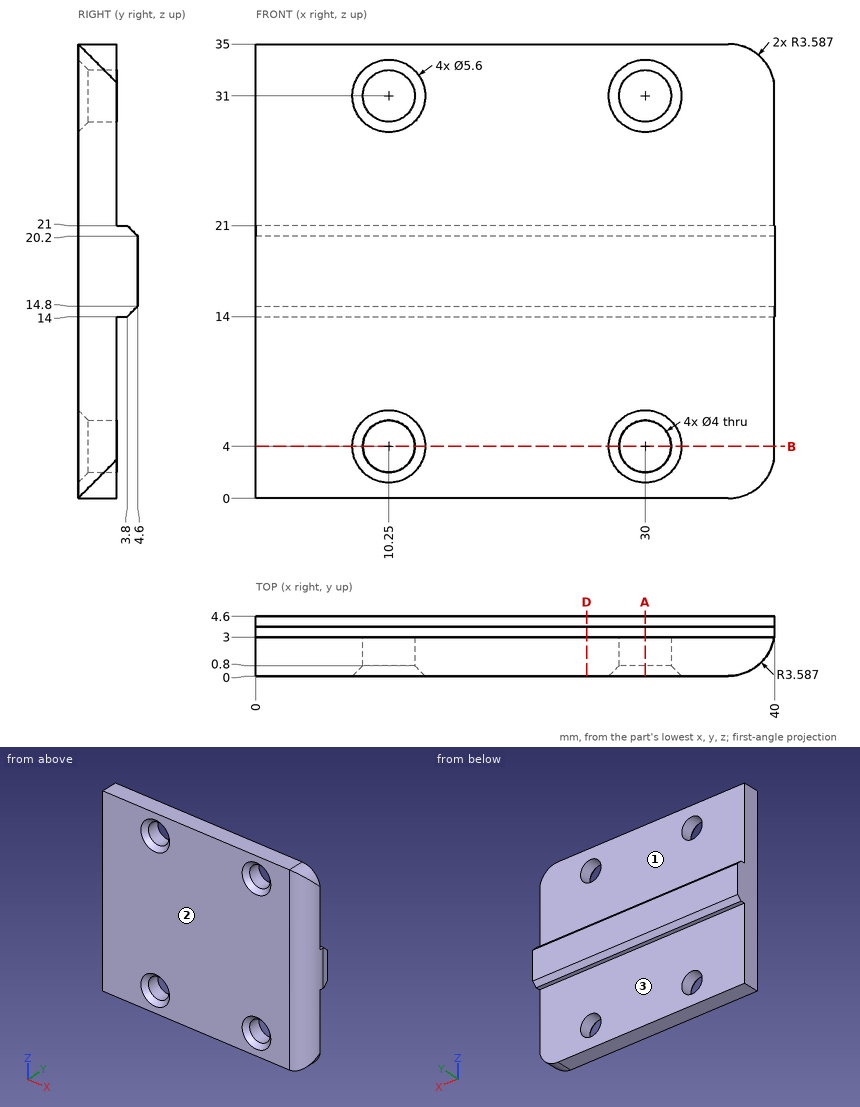
Geometry: see drawing. Coordinates: mm, zero at the bounding-box minimum. A direction names the side the tool comes from. Round coordinates to 2 decimals unless told otherwise and drop trailing zeros. Loops run counter-clockwise (first coordinate to the right, second up) from the corner with the lowest first, then second, coordinate; pieces in that order, holes last. Notation, with made-up numbers: M 41.5,89 L 69.5,89 A21 cw 69.5,115 Z; hole C 53,34 d8. An arc over 180 degrees is marked long. Use a Markdown table: item, result. Add a question column.
1. Cut plane D-D, the plane x = 25.5. Output: boundary loops of the cut face in (y, z).
2. Contact query for flat-ended pins moving along their axis: pin 1 (4.5 mm diameter, centred on x = 30, z = 4, fed in from +Y); pin 2 (2 mm diameter, centred on x = 7.5, y = 1.5, fed in from -Z); pin 3 (3.5 mm diameter, centred on x = 10.25, z = 4, fed in from +Y); pin 4 (2 mm diameter, centred on y = 1.5, z = 5, fed in from +X). Output: stop coordinate, or through.
3. Cut plane B-B, the plane z = 4. State how many separate pieces and enclosed holes the cut face has.
4. Cut plane A-A, the plane x = 30. Output: boundary loops of the cut face in (y, z).
5. Ray query, line 1 along Z through (x, y) = (10.25, 2.3); line 2 along X through (y, z) = (2, 31); line 3 along X through (y, z) = (2.3, 31). Return the intervals inside material, ascending. Write a range as [from, to].
6. Set-up query: the marked faces 1, 2 and 3. Return all of +Z, -Z, +X, -X, +Y, -Y with unobstructed straight access to the full face (end or side cutting, diameter ignored); none if empty.
Solution:
| question | item | result |
|---|---|---|
| 1 | outline | M 0,0 L 3,0 L 3,14 L 3.8,14 L 4.6,14.8 L 4.6,20.2 L 3.8,21 L 3,21 L 3,35 L 0,35 Z |
| 2 | pin 1 | stops at y = 3 |
| 2 | pin 2 | stops at z = 0 |
| 2 | pin 3 | passes through |
| 2 | pin 4 | stops at x = 39.83 |
| 3 | separate pieces | 3 |
| 3 | enclosed holes | 0 |
| 4 | outline | M 0,0 L 3,0 L 3,2 L 0.8,2 L 0,1.2 Z; M 0,6.8 L 0.8,6 L 3,6 L 3,14 L 3.8,14 L 4.6,14.8 L 4.6,20.2 L 3.8,21 L 3,21 L 3,29 L 0.8,29 L 0,28.2 Z; M 0,33.8 L 0.8,33 L 3,33 L 3,35 L 0,35 Z |
| 5 | line 1 | z = [0, 2], [6, 29], [33, 35] |
| 5 | line 2 | x = [0, 8.25], [12.25, 28], [32, 39.63] |
| 5 | line 3 | x = [0, 8.25], [12.25, 28], [32, 39.76] |
| 6 | face 1 | +Z, +X, -X, +Y |
| 6 | face 2 | +Z, -Z, +X, -X, -Y |
| 6 | face 3 | -Z, +X, -X, +Y |
